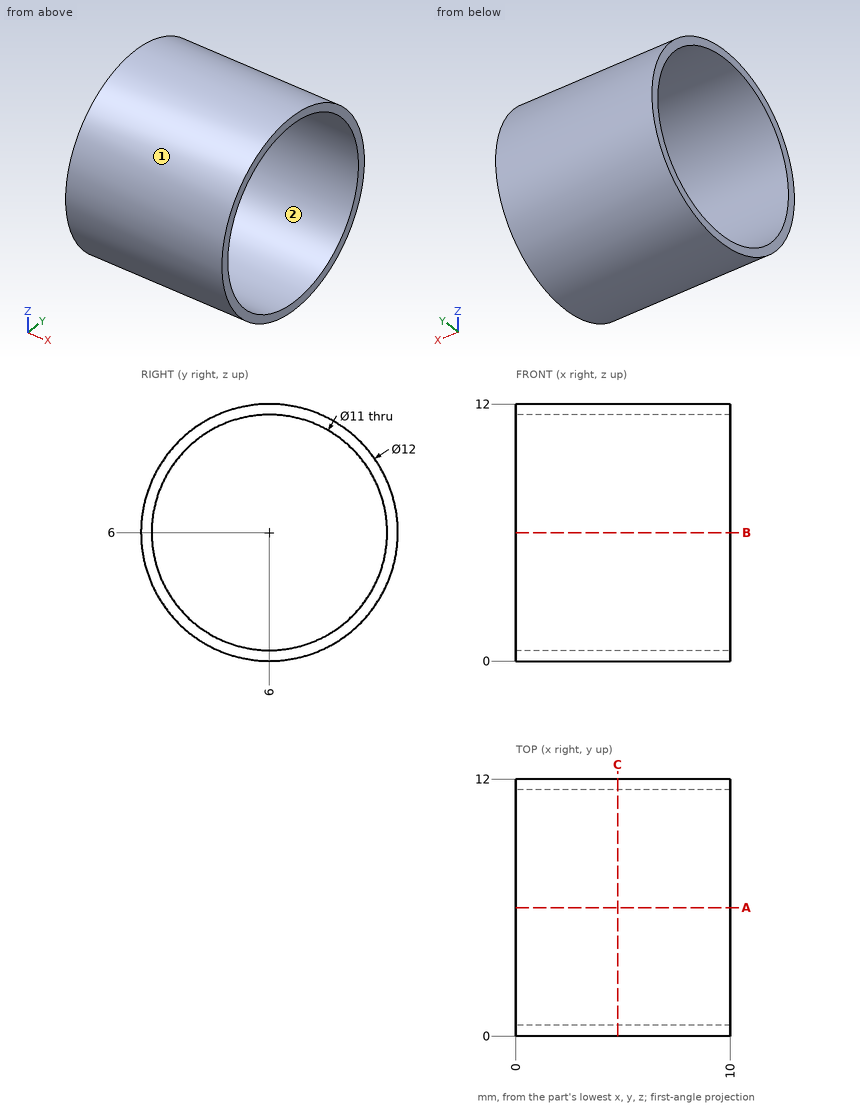
The drawing under review shows one solid part. Ordinate dimensions are in mm from its lowest x, y, z. Round coordinates to 2 decimals unless told otherwise and drop trailing zeros. Loops run counter-clockwise (first coordinate to the right, second up) from the corner with the lowest first, then second, coordinate; pieces in that order, holes last.
Item 1: Clearance check with flat-ended pins moving along their axes: pin 1 Ø5 at (y, z) = (4, 2.5) entering from -X; pin 2 Ø2 at (x, z) = (3.5, 8) entering from -Y. State where each tip first meets the part, or that it passes through.
Determined:
pin 1: stops at x = 0
pin 2: stops at y = 0.08
Item 2: For line 1 (Y direction, x = 4, z = 6); line 2 (Z direction, x = 8.75, y = 9); line 3 (Z direction, x = 4, y = 3.5), list the stretches that pass through material, from the lowest coordinate up.
Determined:
line 1: y = 0 to 0.5, 11.5 to 12
line 2: z = 0.8 to 1.39, 10.61 to 11.2
line 3: z = 0.55 to 1.1, 10.9 to 11.45
Item 3: Take a section at C-C (x = 4.75). Write out the cut boundary in (y, z).
Determined:
outline: circle Ø12 at (6, 6); hole circle Ø11 at (6, 6)
Item 4: Mouldability with a two-part tool opening along Y and no side actions: class the marked faces 1 and 2 as released by +Y, released by -Y, zero draft, split by the parting line, or undercut.
Determined:
face 1: split by the parting line
face 2: undercut
Item 5: Take a section at A-A (y = 6). Write out the cut boundary in (x, z), then the cut area to 3 significant figures.
Determined:
outline: (0, 0) - (10, 0) - (10, 0.5) - (0, 0.5) - close; (0, 11.5) - (10, 11.5) - (10, 12) - (0, 12) - close
area: 10.0 mm2
